from build123d import *

# Parameters (mm, degrees)
SKETCH1_W               = 60
SKETCH1_H               = 35
BOSS_EXTRUDE1_DEPTH     = 8
CUT_EXTRUDE1_DEPTH      = 1
CUT_EXTRUDE1_DEPTH_BACK = 61
FILLET1_R               = 2
SKETCH3_W               = 22
SKETCH3_H               = 2
CUT_EXTRUDE2_DEPTH      = 36
SKETCH5_W               = 35
SKETCH5_H               = 2
BOSS_EXTRUDE2_DEPTH     = 10


with BuildPart() as part:
    # Sketch1 → Boss-Extrude1 (new body)
    with BuildSketch(Plane(origin=(0, 0, 0), x_dir=(1, 0, 0), z_dir=(0, 1, 0))):
        Rectangle(SKETCH1_W, SKETCH1_H)
    extrude(amount=-BOSS_EXTRUDE1_DEPTH)

    # Sketch2 → Cut-Extrude1 (cut, two sides)
    with BuildSketch(Plane(origin=(30, 0, 0), x_dir=(0, 0, -1), z_dir=(1, 0, 0))) as cut_extrude1_sk:
        Polygon((-12.5, -5), (-17.5, -8), (0, -8), (0, -5), align=None)
        Polygon((0, -5), (0, -8), (17.5, -8), (12.5, -5), align=None)
    extrude(amount=CUT_EXTRUDE1_DEPTH, mode=Mode.SUBTRACT)
    extrude(cut_extrude1_sk.sketch, amount=-CUT_EXTRUDE1_DEPTH_BACK, mode=Mode.SUBTRACT)

    # Fillet1
    fillet1_edges = [part.edges().sort_by_distance(p)[0] for p in [
        (0, -8, -17.5),
        (0, -5, 12.5),
        (0, -5, -12.5),
        (0, -8, 17.5),
    ]]
    fillet(fillet1_edges, radius=FILLET1_R)

    # Sketch3 → Cut-Extrude2 (cut, through all)
    with BuildSketch(Plane.XY.offset(17.5)):
        with Locations((-15, -1)):
            Rectangle(SKETCH3_W, SKETCH3_H)
        with Locations((15, -1)):
            Rectangle(SKETCH3_W, SKETCH3_H)
    extrude(amount=-CUT_EXTRUDE2_DEPTH, mode=Mode.SUBTRACT)

    # Sketch5 → Boss-Extrude2 (add)
    with BuildSketch(Plane.ZY.offset(30)):
        with Locations((0, -1)):
            Rectangle(SKETCH5_W, SKETCH5_H)
    boss_extrude2 = extrude(amount=BOSS_EXTRUDE2_DEPTH)

    # Mirror1: Boss-Extrude2 across plane
    add(boss_extrude2.mirror(Plane(origin=(0, 0, 0), x_dir=(0, 0, 1), z_dir=(1, 0, 0))))


solid = part.part
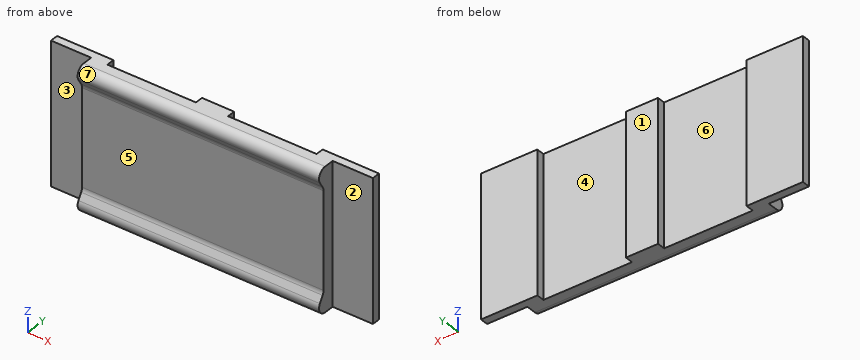
Build history of the part. All positions in model axes, mm. Face numbers are marked on the shaded views. A direction names the side the tool comes from. Coordinates: 2 decimals unless noted, no trailing zeros. Write each loop counter-clockwise with the first axis right and the second up, starting at its lowest first coordinate (ties: lowest second). Pieces come first, ordered by that corner, then holes. Notation, with made-up numbers: (30.25, -4.5) -> (76.25, -4.5) arc R25 cw to (76.25, 34.5) -> close; hole circle Ø1 at (81.5, -17.75). An arc over 180 degrees is marked (long way). Use CSV: the item, a comma, the result in double quotes. Start each with the question number.
Q1. Cut at B-B, the plane x = 0. List the corners of the cut face in (y, z), then the cut area to 3 significant figures.
Q2. Pull direction Z, two halves, no side cores. Call the marked faces 6 and 7: released by +Z, released by -Z, zero draft, split by the parting line, or undercut.
Q3. Cut at A-A, the plane y = -1.25. List the corners of the cut face in (x, z), then the cut area to 3 significant figures.
Q4. Drill centre lines: probe 1 along X at (y, z) = (-0.25, -10); probe 2 along Y at (x, z) = (-2.5, -6.5); probe 3 along X at (y, z) = (-4.25, 0). Where is each one in solid material? Low to high.
Q5. Flat gauge pins, fed straight in: pin 1 Ø6.5 at (x, z) = (-11, 3) entering from +Y; pin 2 Ø3 at (x, z) = (33.5, 6.5) entering from -Y; pin 3 Ø1 at (x, z) = (23.5, -8.5) entering from -Y. Where does each tip first touch, or does it go through?
Q6. Cut at C-C, the plane z = 7.5. List the corners of the cut face in (x, y), then the cut area to 3 significant figures.
Q7. 3-axis set-ups, long thin cutter, end or side, ignore diameter. For the marked faces 1, 2, 3, 4 and 5: which of +Z, -Z, +X, -X, +Y, -Y reach the whole face in a straight line?
Q8. Cut at D-D, the plane x = 35.5. List the corners of the cut face in (y, z), then the cut area to 3 significant figures.
Checked values:
1,outline,"(-6.18, -14.47) arc R2 ccw to (-4.47, -17.5) -> (0, -17.5) -> (0, 17.5) -> (-4.47, 17.5) arc R2 ccw to (-6.18, 14.47) -> (-5.29, 12.98) arc R2 cw to (-5, 11.95) -> (-5, -11.95) arc R2 cw to (-5.29, -12.98) -> close"
1,area,"184 mm²"
2,face 6,"zero draft"
2,face 7,"undercut"
3,outline,"(-40, -17.5) -> (-26, -17.5) -> (-26, 17.5) -> (-40, 17.5) -> close; (-4, -17.5) -> (4, -17.5) -> (4, 17.5) -> (-4, 17.5) -> close; (26, -17.5) -> (40, -17.5) -> (40, 17.5) -> (26, 17.5) -> close"
3,area,"1,260 mm²"
4,probe 1,"x = -40 to -26, -4 to 4, 26 to 40"
4,probe 2,"y = -5 to 0"
4,probe 3,"x = -30 to 30"
5,pin 1,"stops at y = -2"
5,pin 2,"stops at y = -2"
5,pin 3,"stops at y = -5"
6,outline,"(-40, -2) -> (-30, -2) -> (-30, -5) -> (30, -5) -> (30, -2) -> (40, -2) -> (40, 0) -> (26, 0) -> (26, -2) -> (4, -2) -> (4, 0) -> (-4, 0) -> (-4, -2) -> (-26, -2) -> (-26, 0) -> (-40, 0) -> close"
6,area,"252 mm²"
7,face 1,"+Z, -Z, +X, -X, +Y"
7,face 2,"+Z, -Z, +X, -Y"
7,face 3,"+Z, -Z, -X, -Y"
7,face 4,"+Z, -Z, +Y"
7,face 5,"+X, -X, -Y"
8,outline,"(-2, -17.5) -> (0, -17.5) -> (0, 17.5) -> (-2, 17.5) -> close"
8,area,"70.0 mm²"
